Model file for the job. Use its own axes, mm. Face numbers are marked on the shaded views. A direction names the side the tool comes from. Round coordinates to 2 decimals unless told otherwise and drop trailing zeros. Order: outer loops, then holes, each group sorted by start corner. A loop starts at its lowest first (then second) coordinate and runs counter-clockwise, first axis right, second up. Notation, with made-up numbers: (76.5, -37) - (135.5, -37) arc R21 cw to (135.5, 0) - close; hole circle Ø7 at (78.5, 47). An arc over 180 degrees is marked (long way). Write item = value, one per line.
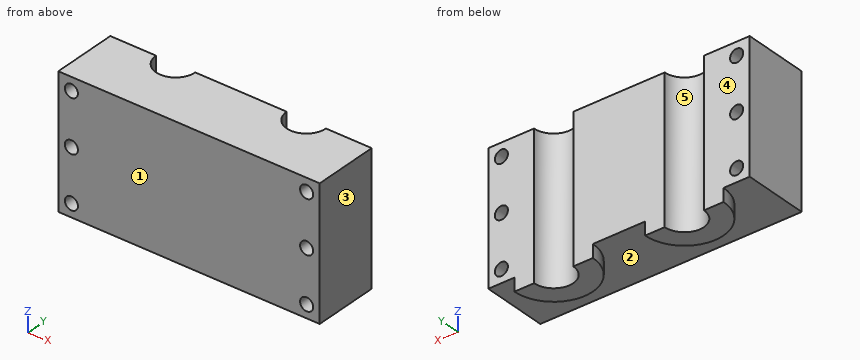
```python
from build123d import *

# Parameters (mm, degrees)
SKETCH1_R               = 6.350000000000003
SKETCH1_R_2             = 6.349999999999967
SKETCH1_R_3             = 6.3499999999999375
SKETCH1_R_4             = 6.349999999999968
SKETCH1_R_5             = 6.350000000000001
SKETCH1_R_6             = 6.35000000000001
BOSS_EXTRUDE3_DEPTH     = 63.5
BOSS_EXTRUDE9_DEPTH     = 12.7
CUT_EXTRUDE5_DEPTH      = 291.99355662969583
CUT_EXTRUDE5_DEPTH_BACK = 291.99355662969583


with BuildPart() as part:
    # Sketch1 → Boss-Extrude3 (new body)
    with BuildSketch(Plane(origin=(0, 0, 0), x_dir=(1, 0, 0), z_dir=(0, 1, 0))):
        Polygon((0, 0), (254, 0), (254, -127), (1.555e-14, -127), align=None)
        with Locations(Location((12.69999999999899, -12.700000000000003, 0), (0, 0, 270))):
            Circle(SKETCH1_R, mode=Mode.SUBTRACT)
        with Locations(Location((241.299999999999, -12.700000000000003, 0), (0, 0, 270))):
            Circle(SKETCH1_R_2, mode=Mode.SUBTRACT)
        with Locations(Location((241.29999999999953, -63.5, 0), (0, 0, 270))):
            Circle(SKETCH1_R_3, mode=Mode.SUBTRACT)
        with Locations(Location((241.30000000000004, -114.3, 0), (0, 0, 270))):
            Circle(SKETCH1_R_4, mode=Mode.SUBTRACT)
        with Locations(Location((12.699999999999523, -63.5, 0), (0, 0, 270))):
            Circle(SKETCH1_R_5, mode=Mode.SUBTRACT)
        with Locations(Location((12.700000000000053, -114.3, 0), (0, 0, 270))):
            Circle(SKETCH1_R_6, mode=Mode.SUBTRACT)
    extrude(amount=BOSS_EXTRUDE3_DEPTH)

    # Sketch3 → Boss-Extrude9 (add)
    with BuildSketch(Plane(origin=(0, 0, 0), x_dir=(-1, 0, 0), z_dir=(0, 0, -1))):
        with BuildLine():
            ThreePointArc((-228.6, 63.5), (-190.5, 25.400000000000013), (-152.4, 63.49999999999999))
            Line((-152.4, 63.5), (-171.45, 63.5))
            ThreePointArc((-171.45, 63.5), (-190.5, 44.44999999999999), (-209.55, 63.5))
            Line((-209.55, 63.5), (-228.6, 63.5))
        make_face()
        with BuildLine():
            Line((-82.55000000000001, 63.5), (-101.6, 63.5))
            ThreePointArc((-101.6, 63.49999999999999), (-63.5, 25.400000000000006), (-25.400000000000006, 63.5))
            Line((-25.400000000000006, 63.5), (-44.44999999999999, 63.5))
            ThreePointArc((-44.44999999999999, 63.5), (-63.5, 44.44999999999999), (-82.55000000000001, 63.5))
        make_face()
    extrude(amount=BOSS_EXTRUDE9_DEPTH)

    # Sketch3_12 → Cut-Extrude5 (cut, two sides: drawn at the far end of the back side and taken through both)
    with BuildSketch(Plane(origin=(0, 0, 0), x_dir=(-1, 0, 0), z_dir=(0, 0, -1)).offset(-CUT_EXTRUDE5_DEPTH_BACK)):
        with BuildLine():
            Line((-44.44999999999999, 63.5), (-82.55000000000001, 63.5))
            ThreePointArc((-82.55000000000001, 63.5), (-63.5, 44.44999999999999), (-44.44999999999999, 63.5))
        make_face()
        with BuildLine():
            ThreePointArc((-209.55, 63.5), (-190.5, 44.44999999999999), (-171.45, 63.5))
            Line((-171.45, 63.5), (-209.55, 63.5))
        make_face()
    extrude(amount=CUT_EXTRUDE5_DEPTH + CUT_EXTRUDE5_DEPTH_BACK, mode=Mode.SUBTRACT)


solid = part.part
```
1) Flat gauge pins, fed straight in: pin 1 Ø11.5 at (x, z) = (241.3, 12.7) entering from -Y; pin 2 Ø1 at (x, z) = (204.5, 101) entering from +Y. Where does each tip first touch, or does it go through?
Conclusion:
pin_1 = through
pin_2 = 51.14
2) Cut at D-D (y = 57). Give the number of separate pieces and of enclosed holes in the cut face, and give its area (3 significant figures).
Conclusion:
separate_pieces = 3
enclosed_holes = 6
area = 23,400 mm^2
3) Cut at B-B (z = 63.5). Write the cut outline in (x, y), and give its area (3 significant figures).
Conclusion:
outline = (0, 0) - (6.35, 0) - (6.35, 63.5) - (0, 63.5) - close; (19.05, 0) - (234.95, 0) - (234.95, 63.5) - (209.55, 63.5) arc R19.05 cw to (171.45, 63.5) - (82.55, 63.5) arc R19.05 cw to (44.45, 63.5) - (19.05, 63.5) - close; (247.65, 0) - (254, 0) - (254, 63.5) - (247.65, 63.5) - close
area = 13,400 mm^2
4) Wall check: line 1 along X through (y, z) = (34, 114.3); line 2 along Z through (x, y) = (12, 11.5); line 3 along Z through (x, y) = (40, 16.5). Give the ranges that are in metal, low to high.
Conclusion:
line_1 = 0 to 6.35, 19.05 to 234.95, 247.65 to 254
line_2 = 0 to 6.39, 19.01 to 57.19, 69.81 to 107.99, 120.61 to 127
line_3 = 0 to 127
5) 3-axis set-ups, long thin cutter, end or side, ignore diameter. For the marked faces 1 and 2: which of +Z, -Z, +X, -X, +Y, -Y reach the whole face in a straight line?
Conclusion:
face_1 = +Z, -Z, +X, -X, -Y
face_2 = -Z, -Y
6) Cut at A-A (x = 241.3). Write the cut outline in (y, z).
Conclusion:
outline = (0, 0) - (63.5, 0) - (63.5, 6.35) - (0, 6.35) - close; (0, 19.05) - (63.5, 19.05) - (63.5, 57.15) - (0, 57.15) - close; (0, 69.85) - (63.5, 69.85) - (63.5, 107.95) - (0, 107.95) - close; (0, 120.65) - (63.5, 120.65) - (63.5, 127) - (0, 127) - close
7) Cut at C-C (y = 17). Write the cut outline in (x, z).
Conclusion:
outline = (0, 0) - (254, 0) - (254, 127) - (0, 127) - close; hole circle Ø12.7 at (12.7, 12.7); hole circle Ø12.7 at (12.7, 63.5); hole circle Ø12.7 at (12.7, 114.3); hole circle Ø12.7 at (241.3, 12.7); hole circle Ø12.7 at (241.3, 63.5); hole circle Ø12.7 at (241.3, 114.3)
8) Mould opens along X. For the marked faces 3, 4 and 5 say: +X half, -X half, draft (parallel to the pull), parting line (faces both ways), or undercut.
Conclusion:
face_3 = +X half
face_4 = draft
face_5 = undercut
